```python
from build123d import *

# Parameters (mm, degrees)
BOSS_EXTRUDE1_DEPTH = 10
CUT_EXTRUDE1_DEPTH  = 7
SKETCH3_W           = 15
SKETCH3_H           = 11.874964638
CUT_EXTRUDE2_DEPTH  = 7
CUT_EXTRUDE3_DEPTH  = 7


with BuildPart() as part:
    # Sketch1 → Boss-Extrude1 (new body)
    with BuildSketch(Plane.XY):
        Polygon((-28.187365871, 32.751649119), (21.812634129, 32.751649119), (21.812634129, -27.017852667), (-28.187365871, -27.017852667), (-38.187365871, -27.017852667), (-38.187365871, 32.751649119), align=None)
    extrude(amount=BOSS_EXTRUDE1_DEPTH)

    # Sketch2 → Cut-Extrude1 (cut)
    with BuildSketch(Plane.XY.offset(10)):
        with BuildLine():
            Line((-8.298420819, 18.570619113), (14.701579181, 18.570619113))
            ThreePointArc((14.701579181, 18.570619113), (18.237113087, 17.106153019), (19.701579181, 13.570619113))
            Line((19.701579181, 13.570619113), (19.701579181, -10.229380887))
            ThreePointArc((19.701579181, -10.229380887), (18.237113087, -13.764914793), (14.701579181, -15.229380887))
            Line((14.701579181, -15.229380887), (-8.298420819, -15.229380887))
            ThreePointArc((-8.298420819, -15.229380887), (-11.833954725, -13.764914793), (-13.298420819, -10.229380887))
            Line((-13.298420819, -10.229380887), (-13.298420819, 13.570619113))
            ThreePointArc((-13.298420819, 13.570619113), (-11.833954725, 17.106153019), (-8.298420819, 18.570619113))
        make_face()
    extrude(amount=-CUT_EXTRUDE1_DEPTH, mode=Mode.SUBTRACT)

    # Sketch3 → Cut-Extrude2 (cut)
    with BuildSketch(Plane.XY.offset(10)):
        Polygon((5.503263718, 32.751649119), (-2.496736282, 32.751649119), (-2.496736282, 18.570619113), (5.503263718, 18.570619113), (5.503263718, 20.876684481), align=None)
        with Locations((13.003263718, 26.8141668)):
            Rectangle(SKETCH3_W, SKETCH3_H)
    extrude(amount=-CUT_EXTRUDE2_DEPTH, mode=Mode.SUBTRACT)

    # Sketch4 → Cut-Extrude3 (cut)
    with BuildSketch(Plane.XY.offset(10)):
        Polygon((1.563165921, -15.229380887), (7.956099034, -15.229380887), (7.956099034, -24.630130661), (1.563165921, -24.630130661), (-17.923726581, -24.630130661), (-22.688843527, -24.630130661), (-34.888499332, 32.751649119), (-17.923726581, 32.751649119), (-17.923726581, -18.699337291), (1.563165921, -18.699337291), align=None)
    extrude(amount=-CUT_EXTRUDE3_DEPTH, mode=Mode.SUBTRACT)


solid = part.part
```
Work out the finished part from the listing and answer in its coordinate system (mm). A direction names the side the tool comes from. Coordinates: 2 decimals unless noted, no trailing zeros. Write each loop counter-clockwise with the first axis right and the second up, starting at its lowest first coordinate (ties: lowest second). Pieces come first, ordered by that corner, then holes. Notation, with made-up numbers: (63, 41.5) - (85, 41.5) arc R29 cw to (85, 64.5) - close; hole circle Ø7 at (60, 42). An arc over 180 degrees is marked (long way). Answer as a JSON object with one key per item and string values.
Q1. Find section A-A (z = 4.5). Write down the section's boundary in (x, y), plus the area to 3 significant figures.
Results list:
{"outline": "(-38.19, -27.02) - (21.81, -27.02) - (21.81, 32.75) - (20.5, 32.75) - (20.5, 20.88) - (5.5, 20.88) - (5.5, 18.57) - (14.7, 18.57) arc R5 cw to (19.7, 13.57) - (19.7, -10.23) arc R5 cw to (14.7, -15.23) - (7.96, -15.23) - (7.96, -24.63) - (-22.69, -24.63) - (-34.89, 32.75) - (-38.19, 32.75) - close; (-17.92, -18.7) - (1.56, -18.7) - (1.56, -15.23) - (-8.3, -15.23) arc R5 cw to (-13.3, -10.23) - (-13.3, 13.57) arc R5 cw to (-8.3, 18.57) - (-2.5, 18.57) - (-2.5, 32.75) - (-17.92, 32.75) - close", "area": "1,400 mm^2"}
Q2. Consider L1, parallel to Y at x = -4, z = 6.5; L2, parallel to Y at x = 8, z = 5.25; L3, parallel to X at y = 23, z = 4.5. Determine where each line is inside the solid, lowest interval first. Write a range as from..to.
Results list:
{"L1": "y = -27.02..-24.63, -18.7..-15.23, 18.57..32.75", "L2": "y = -27.02..-15.23, 18.57..20.88", "L3": "x = -38.19..-32.82, -17.92..-2.5, 20.5..21.81"}
Q3. Find section D-D (x = -15). Write down the section's boundary in (y, z), plus the area to 3 significant figures.
Results list:
{"outline": "(-27.02, 0) - (32.75, 0) - (32.75, 10) - (-18.7, 10) - (-18.7, 3) - (-24.63, 3) - (-24.63, 10) - (-27.02, 10) - close", "area": "556 mm^2"}
Q4. Given pin 1 Ø3.5 at (x, z) = (10.5, 8) entering from +Y; pin 2 Ø10 at (x, y) = (14, -10) entering from +Z; pin 3 Ø1 at (x, y) = (13, -15) entering from +Z, each flat-ended and moving along its own axis, determine where each tip first touches the part or whether it passes through.
Results list:
{"pin 1": "stops at y = 20.88", "pin 2": "stops at z = 3", "pin 3": "stops at z = 10"}
Q5. Find section C-C (y = -12.5). Write down the section's boundary in (x, z), plus the area to 3 significant figures.
Results list:
{"outline": "(-38.19, 0) - (21.81, 0) - (21.81, 10) - (19.16, 10) - (19.16, 3) - (-12.75, 3) - (-12.75, 10) - (-17.92, 10) - (-17.92, 3) - (-25.27, 3) - (-25.27, 10) - (-38.19, 10) - close", "area": "325 mm^2"}
Q6. Find section B-B (x = 9). Write down the section's boundary in (y, z), plus the area to 3 significant figures.
Results list:
{"outline": "(-27.02, 0) - (32.75, 0) - (32.75, 3) - (20.88, 3) - (20.88, 10) - (18.57, 10) - (18.57, 3) - (-15.23, 3) - (-15.23, 10) - (-27.02, 10) - close", "area": "278 mm^2"}
Q7. Which of the six approach directions +Z, -Z, +X, -X, +Y, -Y give full straight-line access (tool end or side, diameter ignored) to faces 5 (the flat face through (-2.497, 26, 7)), 6 (the flat face through (10, 18.571, 7)), 7 (the flat face through (-26, -10, 10))?
Results list:
{"face 5": "+Z, +Y", "face 6": "+Z", "face 7": "+Z, +X, -X, +Y, -Y"}
Q8. For a pull along Y with two mould halves and no side action, classify faces 1 (the flat face through (-8, -24.63, 7)), 2 (the flat face through (-9, -27.018, 5)), 3 (the flat face through (-15, 7, 10)), 4 (the flat face through (-28.703, 3.659, 6.549)) as pulls with the +Y half, pulls with the -Y half, needs draft (parallel to the pull), parting line crosses it, or undercut.
Results list:
{"face 1": "undercut", "face 2": "pulls with the -Y half", "face 3": "needs draft", "face 4": "pulls with the +Y half"}
